Here's how the part is built. I have some questions about the finished solid (model axes, mm). A direction names the side the tool comes from. Round coordinates to 2 decimals unless told otherwise and drop trailing zeros. Loops run counter-clockwise (first coordinate to the right, second up) from the corner with the lowest first, then second, coordinate; pieces in that order, holes last. Notation, with made-up numbers: M 3.5,56 L 38.5,56 A12 ccw 38.5,73 Z; hole C 15.5,-26 d2. An arc over 180 degrees is marked long. Put each result on its own line as item: value. Start each with the question number.
```python
from build123d import *

# Parameters (mm, degrees)
BOSS_EXTRUDE1_DEPTH      = 15
BOSS_EXTRUDE2_DEPTH      = 66
CUT_EXTRUDE1_DEPTH       = 16
FILLET1_R                = 0.2
SKETCH5_R                = 32.25
CUT_EXTRUDE2_DEPTH       = 66
BOSS_EXTRUDE7_DEPTH      = 7
BOSS_EXTRUDE9_DEPTH      = 13.5
BOSS_EXTRUDE9_DEPTH_BACK = 7
BOSS_EXTRUDE10_DEPTH     = 5


with BuildPart() as part:
    # Sketch1 → Boss-Extrude1 (new body)
    with BuildSketch(Plane.XY):
        with BuildLine():
            Line((-35.569135578, 10.252622841), (-35.569135578, 6.252622841))
            Line((-35.569135578, 6.252622841), (-34.569135578, 6.252622841))
            Line((-34.569135578, 6.252622841), (-34.569135578, -0.747377159))
            ThreePointArc((-34.569135578, -0.747377159), (-33.104669484, -4.282911065), (-29.569135578, -5.747377159))
            Line((-29.569135578, -5.747377159), (28.430864422, -5.747377159))
            ThreePointArc((28.430864422, -5.747377159), (31.966398327, -4.282911065), (33.430864422, -0.747377159))
            Line((33.430864422, -0.747377159), (33.430864422, 6.252622841))
            Line((33.430864422, 6.252622841), (33.930864422, 10.252622841))
            Line((33.930864422, 10.252622841), (30.930864422, 10.252622841))
            Line((30.930864422, 10.252622841), (30.930864422, 1.252622841))
            ThreePointArc((30.930864422, 1.252622841), (29.759291546, -1.575804284), (26.930864422, -2.747377159))
            Line((26.930864422, -2.747377159), (-28.569135578, -2.747377159))
            ThreePointArc((-28.569135578, -2.747377159), (-31.397562703, -1.575804284), (-32.569135578, 1.252622841))
            Line((-32.569135578, 1.252622841), (-32.569135578, 10.252622841))
            Line((-32.569135578, 10.252622841), (-35.569135578, 10.252622841))
        make_face()
    boss_extrude1 = extrude(amount=BOSS_EXTRUDE1_DEPTH)

    # Sketch2 → Boss-Extrude2 (add)
    with BuildSketch(Plane.XY.offset(15)):
        Polygon((33.430864422, -5.747377159), (-34.569135578, -5.747377159), (-34.569135578, 10.252622841), (-32.569135578, 10.252622841), (-32.569135578, -2.747377159), (30.930864422, -2.747377159), (30.930864422, 10.252622841), (33.430864422, 10.252622841), align=None)
    extrude(amount=BOSS_EXTRUDE2_DEPTH)

    # Mirror1: Boss-Extrude1 across plane
    add(boss_extrude1.mirror(Plane(origin=(0, 0, 48), x_dir=(1, 0, 0), z_dir=(0, 0, -1))))

    # Sketch4 → Cut-Extrude1 (cut)
    with BuildSketch(Plane.XZ.offset(5.747377159)):
        Polygon((-34.569135578, 15), (-27.069135578, 15), (-34.569135578, 18.37), align=None)
        Polygon((33.430864422, 18.37), (33.430864422, 15), (25.930864422, 15), align=None)
        Polygon((33.430864422, 81), (25.930864422, 81), (33.430864422, 77.63), align=None)
        Polygon((-34.569135578, 77.63), (-34.569135578, 81), (-27.069135578, 81), align=None)
    extrude(amount=-CUT_EXTRUDE1_DEPTH, mode=Mode.SUBTRACT)

    # Fillet1
    fillet1_edges = [part.edges().sort_by_distance(p)[0] for p in [
        (-27.069135578, -4.247377159, 15),
        (25.930864422, -4.247377159, 15),
        (25.930864422, -4.247377159, 81),
        (-27.069135578, -4.247377159, 81),
    ]]
    fillet(fillet1_edges, radius=FILLET1_R)

    # Sketch5 → Cut-Extrude2 (cut)
    with BuildSketch(Plane.XZ.offset(5.747377159)):
        with Locations((-0.569135578, 48)):
            Circle(SKETCH5_R)
    extrude(amount=-CUT_EXTRUDE2_DEPTH, mode=Mode.SUBTRACT)

    # Sketch14 → Boss-Extrude7 (add)
    with BuildSketch(Plane.XZ.offset(5.747377159)):
        with BuildLine():
            Line((-10.647665103, 80.175600928), (-10.647665103, 78.600128297))
            ThreePointArc((-10.647665103, 78.600128297), (-32.786283329, 48), (-10.647665103, 17.399871703))
            Line((-10.647665103, 17.399871703), (-10.647665103, 15.824399072))
            ThreePointArc((-10.647665103, 15.824399072), (-34.286283329, 48), (-10.647665103, 80.175600928))
        make_face()
        with BuildLine():
            Line((9.509393946, 17.399871703), (9.509393946, 15.824399072))
            ThreePointArc((9.509393946, 15.824399072), (33.148012172, 48), (9.509393946, 80.175600928))
            Line((9.509393946, 80.175600928), (9.509393946, 78.600128297))
            ThreePointArc((9.509393946, 78.600128297), (31.648012172, 48), (9.509393946, 17.399871703))
        make_face()
    extrude(amount=BOSS_EXTRUDE7_DEPTH)

    # Sketch15 → Boss-Extrude9 (add, two sides)
    with BuildSketch(Plane.XZ.offset(12.747377159)) as boss_extrude9_sk:
        with BuildLine():
            Line((-28.026086912, 70.843608886), (-25.530250363, 68.367592208))
            ThreePointArc((-25.530250363, 68.367592208), (-23.518464715, 70.610271024), (-21.305976378, 72.655212375))
            Line((-21.305976378, 72.655212375), (-23.798751135, 75.131155606))
            ThreePointArc((-23.798751135, 75.131155606), (-26.002927667, 73.076619857), (-28.026086912, 70.843608886))
        make_face()
        with BuildLine():
            Line((22.660479978, 75.131155606), (20.167705221, 72.655212375))
            ThreePointArc((20.167705221, 72.655212375), (22.380193558, 70.610271024), (24.391979206, 68.367592208))
            Line((24.391979206, 68.367592208), (26.887815755, 70.843608886))
            ThreePointArc((26.887815755, 70.843608886), (24.86465651, 73.076619857), (22.660479978, 75.131155606))
        make_face()
        with BuildLine():
            Line((19.996816858, 23.202063312), (22.492653407, 20.726046634))
            ThreePointArc((22.492653407, 20.726046634), (24.694346544, 22.751809679), (26.718776146, 24.954728963))
            Line((26.718776146, 24.954728963), (24.212854805, 27.414835044))
            ThreePointArc((24.212854805, 27.414835044), (22.202466054, 25.210743262), (19.996816858, 23.202063312))
        make_face()
        with BuildLine():
            Line((-21.135088015, 23.202063312), (-23.630924564, 20.726046634))
            ThreePointArc((-23.630924564, 20.726046634), (-25.832617701, 22.751809679), (-27.857047303, 24.954728963))
            Line((-27.857047303, 24.954728963), (-25.351125962, 27.414835044))
            ThreePointArc((-25.351125962, 27.414835044), (-23.340737211, 25.210743262), (-21.135088015, 23.202063312))
        make_face()
    extrude(amount=BOSS_EXTRUDE9_DEPTH)
    extrude(boss_extrude9_sk.sketch, amount=-BOSS_EXTRUDE9_DEPTH_BACK)

    # Sketch17 → Boss-Extrude10 (add)
    with BuildSketch(Plane.XZ.offset(26.247377159)):
        with BuildLine():
            Line((-8.787404877, 35.45169136), (-23.630924564, 20.726046634))
            ThreePointArc((-23.630924564, 20.726046634), (-25.832617701, 22.751809679), (-27.857047303, 24.954728963))
            Line((-27.857047303, 24.954728963), (-12.973551792, 39.566112498))
            ThreePointArc((-12.973551792, 39.566112498), (-15.567939739, 47.810596324), (-13.182567225, 56.11796416))
            Line((-13.182567225, 56.11796416), (-28.026086912, 70.843608886))
            ThreePointArc((-28.026086912, 70.843608886), (-26.002927667, 73.076619857), (-23.798751135, 75.131155606))
            Line((-23.798751135, 75.131155606), (-8.98453465, 60.416966557))
            ThreePointArc((-8.98453465, 60.416966557), (-0.569135578, 63), (7.846263493, 60.416966557))
            Line((7.846263493, 60.416966557), (22.660479978, 75.131155606))
            ThreePointArc((22.660479978, 75.131155606), (24.86465651, 73.076619857), (26.887815755, 70.843608886))
            Line((26.887815755, 70.843608886), (12.044296068, 56.11796416))
            ThreePointArc((12.044296068, 56.11796416), (14.429668582, 47.810596325), (11.835280635, 39.566112498))
            Line((11.835280635, 39.566112498), (26.718776146, 24.954728963))
            ThreePointArc((26.718776146, 24.954728963), (24.694346544, 22.751809679), (22.492653407, 20.726046634))
            Line((22.492653407, 20.726046634), (7.64913372, 35.45169136))
            ThreePointArc((7.64913372, 35.45169136), (-0.569135578, 33), (-8.787404877, 35.45169136))
        make_face()
    extrude(amount=-BOSS_EXTRUDE10_DEPTH)


solid = part.part
```
1) On a 3-axis mill with a long thin cutter (end or side, diameter ignored), from which of +Z, -Z, +X, -X, +Y, -Y can I reach the whole of each face in a straight line? I mean faces 1 (the face through (0, -21.247, 48)), 2 (the face through (-34.569, 2, 48)), 3 (the face through (-16.24, -9.2, 19.85)). Say none if no direction works.
2) Suppose I cut it at A-A (y = -15). Write out the boundary of the cut face in (x, z), plus the area to 3 significant figures.
3) Suppose I cut it at D-D (z = 6). Write out the boundary of the cut face in (x, y).
4) Suppose I cut it at B-B (z = 48). State how many separate pieces and enclosed holes the cut face has, plus the area to 3 significant figures.
5) If we mould it in two halves opening along X, with no side actions, what happens to faces 4 (the face through (24.66, -16.14, 22.72)), 5 (the face through (0, -2.747, 13)), 6 (the face through (-25.8, -16.14, 22.72))? For each: pulls with the +X half, pulls with the -X half, needs draft (parallel to the pull), parting line crosses it, or undercut.
6) If I drill on probe 1 along X at (y, z) = (6, 48); probe 2 along Z at (x, y) = (-26.5, -10); probe 3 along X at (y, z) = (-17, 70), over which ranges is the centre line in solid material (lowest first)? Write a range as from..to.
7) I'm going to push flat-ended pins straight in: P1, Ø4, axis at y = 4.5, z = 66.5, coming from the +X side; P2, Ø8, axis at y = 0.5, z = 38, coming from the -X side; P3, Ø7.5, axis at y = 3, z = 7.5, coming from the +X side. Where does each tip first touch, or does it pass through?
Results are:
1. face 1: +Y
1. face 2: -X, +Y, -Y
1. face 3: +Y, -Y
2. outline: M -28.03,70.84 L -25.53,68.37 A32.22 cw -21.31,72.66 L -23.8,75.13 A35.72 ccw Z; M -27.86,24.95 A35.72 ccw -23.63,20.73 L -21.14,23.2 A32.22 cw -25.35,27.41 Z; M 20,23.2 L 22.49,20.73 A35.72 ccw 26.72,24.95 L 24.21,27.41 A32.22 cw Z; M 20.17,72.66 A32.22 cw 24.39,68.37 L 26.89,70.84 A35.72 ccw 22.66,75.13 Z
2. area: 84.1 mm²
3. outline: M -35.57,6.25 L -34.57,6.25 L -34.57,-0.75 A5 ccw -29.57,-5.75 L 28.43,-5.75 A5 ccw 33.43,-0.75 L 33.43,6.25 L 33.93,10.25 L 30.93,10.25 L 30.93,1.25 A4 cw 26.93,-2.75 L -28.57,-2.75 A4 cw -32.57,1.25 L -32.57,10.25 L -35.57,10.25 Z
4. separate pieces: 3
4. enclosed holes: 0
4. area: 227 mm²
5. face 4: pulls with the +X half
5. face 5: undercut
5. face 6: pulls with the -X half
6. probe 1: -34.57..-32.82, 31.68..33.43
6. probe 2: 23.44..26.29, 26.45..28.88, 67.12..72.56
6. probe 3: -27.18..-24.1, 22.97..26.04
7. P1: x = 33.43
7. P2: x = -34.57
7. P3: x = 33.49
